```python
from build123d import *

# Parameters (mm, degrees)
SKETCH_1_W          = 28
SKETCH_1_H          = 28
SKETCH_1_R          = 2.5
SKETCH_1_R_2        = 5
EXTRUDE_1_DEPTH     = 6
SKETCH_2_R          = 1.5
CUT_EXTRUDE_1_DEPTH = 32.874754901
CHAMFER_2_SIZE      = 1
SKETCH_8_W          = 28
SKETCH_8_H          = 0.1
EXTRUDE_4_DEPTH     = 6
SKETCH_9_W          = 28
SKETCH_9_H          = 0.1
CUT_EXTRUDE_4_DEPTH = 21.755962999
SKETCH_10_R         = 1.5
CUT_EXTRUDE_5_DEPTH = 32.874754901
CUT_EXTRUDE_START   = -3
SKETCH_11_W         = 9
SKETCH_11_H         = 10
SKETCH_11_R         = 1.5
CUT_EXTRUDE_6_DEPTH = 3
SKETCH_12_W         = 9
SKETCH_12_H         = 9
SKETCH_12_R         = 1.5
CUT_EXTRUDE_7_DEPTH = 3
FILLET_1_R          = 3


with BuildPart() as part:
    # 草图1 → 凸台-拉伸1 (new body)
    with BuildSketch(Plane.XY):
        Rectangle(SKETCH_1_W, SKETCH_1_H)
        with Locations((0, -6)):
            Circle(SKETCH_1_R, mode=Mode.SUBTRACT)
        with Locations((0, 5.9)):
            Circle(SKETCH_1_R_2, mode=Mode.SUBTRACT)
    extrude(amount=EXTRUDE_1_DEPTH)

    # 草图2 → 切除-拉伸1 (cut, through all)
    with BuildSketch(Plane(origin=(0, -14, 0), x_dir=(-1, 0, 0), z_dir=(0, -1, 0))):
        with Locations(Location((10, -3, 0), (0, 0, 180))):
            Circle(SKETCH_2_R)
        with Locations(Location((-10, -3, 0), (0, 0, 180))):
            Circle(SKETCH_2_R)
    extrude(amount=-CUT_EXTRUDE_1_DEPTH, mode=Mode.SUBTRACT)

    # 倒角2
    chamfer_2_edges = [part.edges().sort_by_distance(p)[0] for p in [
        (-5, 5.9, 0),
    ]]
    chamfer(chamfer_2_edges, length=CHAMFER_2_SIZE)

    # 草图8 → 凸台-拉伸4 (add)
    with BuildSketch(Plane(origin=(0, 0, 0), x_dir=(-1, 0, 0), z_dir=(0, 0, -1))):
        with Locations((0, -14.05)):
            Rectangle(SKETCH_8_W, SKETCH_8_H)
    extrude(amount=-EXTRUDE_4_DEPTH)

    # 草图9 → 切除-拉伸4 (cut, through all)
    with BuildSketch(Plane.XY.offset(6)):
        with Locations((0, 13.95)):
            Rectangle(SKETCH_9_W, SKETCH_9_H)
    extrude(amount=-CUT_EXTRUDE_4_DEPTH, mode=Mode.SUBTRACT)

    # 草图10 → 切除-拉伸5 (cut, through all)
    with BuildSketch(Plane(origin=(0, 13.9, 0), x_dir=(1, 0, 0), z_dir=(0, 1, 0))):
        with Locations(Location((-10, -3, 0), (0, 0, 90))):
            Circle(SKETCH_10_R)
        with Locations(Location((10, -3, 0), (0, 0, 90))):
            Circle(SKETCH_10_R)
    extrude(amount=-CUT_EXTRUDE_5_DEPTH, mode=Mode.SUBTRACT)

    # 草图11 → 切除-拉伸6 (cut)
    # profile 1 of 2: a face of its own
    with BuildSketch(Plane(origin=(0, 13.9, 0), x_dir=(1, 0, 0), z_dir=(0, 1, 0)).offset(CUT_EXTRUDE_START)):
        with Locations((-10, -3)):
            Rectangle(SKETCH_11_W, SKETCH_11_H)
        with Locations(Location((-10, -3, 0), (0, 0, 270))):
            Circle(SKETCH_11_R, mode=Mode.SUBTRACT)
    # profile 2 of 2: a face of its own
    with BuildSketch(Plane(origin=(0, 13.9, 0), x_dir=(1, 0, 0), z_dir=(0, 1, 0)).offset(CUT_EXTRUDE_START)):
        with Locations((10, -3)):
            Rectangle(SKETCH_11_W, SKETCH_11_H)
    extrude(amount=CUT_EXTRUDE_6_DEPTH, mode=Mode.SUBTRACT)

    # 草图12 → 切除-拉伸7 (cut)
    # profile 1 of 2: a face of its own
    with BuildSketch(Plane.XZ.offset(14.1)):
        with Locations((-10, 3)):
            Rectangle(SKETCH_12_W, SKETCH_12_H)
        with Locations(Location((-10, 3, 0), (0, 0, 270))):
            Circle(SKETCH_12_R, mode=Mode.SUBTRACT)
    # profile 2 of 2: a face of its own
    with BuildSketch(Plane.XZ.offset(14.1)):
        with Locations((10, 3)):
            Rectangle(SKETCH_12_W, SKETCH_12_H)
    extrude(amount=-CUT_EXTRUDE_7_DEPTH, mode=Mode.SUBTRACT)

    # 圆角1
    fillet_1_edges = [part.edges().sort_by_distance(p)[0] for p in [
        (5.5, -14.1, 3),
        (-5.5, -14.1, 3),
        (5.5, 13.9, 3),
        (-5.5, 13.9, 3),
    ]]
    fillet(fillet_1_edges, radius=FILLET_1_R - 0.0001)  # a hair under: the kernel refuses the full size


solid = part.part
```
Input: part model. Units: mm. Frame: model coordinates. A direction names the side the tool comes from. Round coordinates to 2 decimals unless told otherwise and drop trailing zeros. Loops run counter-clockwise (first coordinate to the right, second up) from the corner with the lowest first, then second, coordinate; pieces in that order, holes last.
1) Set-up query: faces 1 (the flat face through (8.7, -11.1, 4.4)), 2 (the flat face through (-8.9, -11.1, 4.4)), 3 (the flat face through (8.7, 10.9, 1.6)). Return all of +Z, -Z, +X, -X, +Y, -Y with unobstructed straight access to the full face (end or side cutting, diameter ignored); none if empty.
Ans:
face 1: +Z, -Z, +X, -Y
face 2: +Z, -Z, -X, -Y
face 3: +Z, -Z, +X, +Y
2) Section query A-A on z = 3. Count the separate pieces of the cut face and the enclosed holes in it, plus the area to 3 significant figures.
Ans:
separate pieces: 3
enclosed holes: 2
area: 444 mm2
3) Section query B-B on y = -6. Return the cut outline in (x, z), plus the area to 3 significant figures.
Ans:
outline: (-14, 0) - (-2.5, 0) - (-2.5, 6) - (-14, 6) - close; (2.5, 0) - (14, 0) - (14, 6) - (2.5, 6) - close; hole circle Ø3 at (-10, 3); hole circle Ø3 at (10, 3)
area: 124 mm2
4) Section query C-C on x = 10. Return the cut outline in (y, z), plus the area to 3 significant figures.
Ans:
outline: (-11.1, 0) - (10.9, 0) - (10.9, 1.5) - (-11.1, 1.5) - close; (-11.1, 4.5) - (10.9, 4.5) - (10.9, 6) - (-11.1, 6) - close
area: 66.0 mm2
5) Section query D-D on x = 0. Return the cut outline in (y, z).
Ans:
outline: (-14.1, 0) - (-8.5, 0) - (-8.5, 6) - (-14.1, 6) - close; (-3.5, 0) - (-0.1, 0) - (0.9, 1) - (0.9, 6) - (-3.5, 6) - close; (10.9, 1) - (11.9, 0) - (13.9, 0) - (13.9, 6) - (10.9, 6) - close
6) Pull-direction query (X, two-part tool) for faces 4 (the cylindrical face through (-0.33, -3.52, 2.96)), 5 (the cylindrical face through (4.64, -13.2, 3.04)), 6 (the flat face through (-8.9, 10.9, 1.6)), 7 (the cylindrical face through (-9.31, -0.25, 1.67)); classes: released by +X, released by -X, zero draft, split by the parting line, or undercut.
Ans:
face 4: undercut
face 5: released by +X
face 6: zero draft
face 7: undercut
7) Material intervals for line 1 (Y direction, x = 0, z = 3.6); line 2 (X direction, y = -3.25, z = 2.45); line 3 (Z direction, x = -10, y = 2.75), sorted ascending.
Ans:
line 1: y = -14.1 to -8.5, -3.5 to 0.9, 10.9 to 13.9
line 2: x = -14 to -11.4, -8.6 to 8.6, 11.4 to 14
line 3: z = 0 to 1.5, 4.5 to 6
8) Pin query (flat end, axial travel): pin 1 (2.5 mm diameter, centred on x = 10, z = 3, fed in from -Y); pin 2 (1.8 mm diameter, centred on x = -9, z = 3.5, fed in from -Y); pin 3 (11.5 mm diameter, centred on x = 0, y = 5.9, fed in from -Z). Return the tip coordinate at first contact, or that it passes through.
Ans:
pin 1: passes through
pin 2: stops at y = -11.1
pin 3: stops at z = 0.25
